from build123d import *

# Parameters (mm, degrees)
SKETCH1_R           = 29.337
BOSS_EXTRUDE1_DEPTH = 55.1942
SKETCH2_R           = 10.31875
SKETCH2_R_2         = 9.525
BOSS_EXTRUDE2_DEPTH = 3.175
SKETCH3_R           = 4.0005
BOSS_EXTRUDE3_DEPTH = 34.925
SKETCH4_R           = 2.0193
CUT_EXTRUDE1_DEPTH  = 12.7
CUT_EXTRUDE2_DEPTH  = 5.08
CUT_EXTRUDE3_DEPTH  = 2
FILLET1_R           = 0.127


with BuildPart() as part:
    # Sketch1 → Boss-Extrude1 (new body)
    with BuildSketch(Plane.XY):
        Circle(SKETCH1_R)
    extrude(amount=BOSS_EXTRUDE1_DEPTH)

    # Sketch2 → Boss-Extrude2 (add)
    with BuildSketch(Plane.XY.offset(55.1942)):
        Circle(SKETCH2_R)
        Circle(SKETCH2_R_2, mode=Mode.SUBTRACT)
    extrude(amount=BOSS_EXTRUDE2_DEPTH)

    # Sketch3 → Boss-Extrude3 (add)
    with BuildSketch(Plane.XY.offset(55.1942)):
        Circle(SKETCH3_R)
    extrude(amount=BOSS_EXTRUDE3_DEPTH)

    # Sketch4 → Cut-Extrude1 (cut)
    with BuildSketch(Plane.XY.offset(55.1942)):
        with Locations((17.960512242, -17.960512242)):
            Circle(SKETCH4_R)
        with Locations((-17.960512242, -17.960512242)):
            Circle(SKETCH4_R)
        with Locations((-17.960512242, 17.960512242)):
            Circle(SKETCH4_R)
        with Locations((17.960512242, 17.960512242)):
            Circle(SKETCH4_R)
    extrude(amount=-CUT_EXTRUDE1_DEPTH, mode=Mode.SUBTRACT)

    # Sketch5 → Cut-Extrude2 (cut)
    with BuildSketch(Plane(origin=(0, 29.337, 0), x_dir=(1, 0, 0), z_dir=(0, 1, 0))):
        with BuildLine():
            Line((12.7, -52.0192), (-12.7, -52.0192))
            ThreePointArc((-12.7, -52.0192), (-15.875, -48.8442), (-12.7, -45.6692))
            Line((-12.7, -45.6692), (12.7, -45.6692))
            ThreePointArc((12.7, -45.6692), (15.875, -48.8442), (12.7, -52.0192))
        make_face()
    extrude(amount=-CUT_EXTRUDE2_DEPTH, mode=Mode.SUBTRACT)

    # Sketch6 → Cut-Extrude3 (cut)
    with BuildSketch(Plane(origin=(0, 4.0005, 0), x_dir=(1, 0, 0), z_dir=(0, 1, 0))):
        with BuildLine():
            Line((0.99949, -65.71869), (0.99949, -85.21827))
            ThreePointArc((0.99949, -85.21827), (0, -86.21776), (-0.99949, -85.21827))
            Line((-0.99949, -85.21827), (-0.99949, -65.71869))
            ThreePointArc((-0.99949, -65.71869), (0, -64.7192), (0.99949, -65.71869))
        make_face()
    extrude(amount=-CUT_EXTRUDE3_DEPTH, mode=Mode.SUBTRACT)

    # Fillet1
    fillet1_edges = [part.edges().sort_by_distance(p)[0] for p in [
        (-4.0005, 0, 90.1192),
    ]]
    fillet(fillet1_edges, radius=FILLET1_R)


solid = part.part
Build history of the part. All positions in model axes, mm. A direction names the side the tool comes from. Coordinates: 2 decimals unless noted, no trailing zeros. Order: outer loops, then holes, each group sorted by start corner. A loop starts at its lowest first (then second) coordinate and runs counter-clockwise, first axis right, second up. Notation, with made-up numbers: (74.5, -32.75) - (108.5, -32.75) arc R37 ccw to (108.5, 4.25) - close; hole circle Ø1 at (-37.5, 25). An arc over 180 degrees is marked (long way). Put each result on its own line as item: value.
1. Pull direction Z, two halves, no side cores. Call faces 4 (the face through (17.698, 19.963, 48.933)), 5 (the face through (13, 0, 55.194)), 6 (the face through (-15.7, 24.6, 47.8)): pulls with the +Z half, pulls with the -Z half, needs draft (parallel to the pull), parting line crosses it, or undercut.
Answer sheet:
face 4: needs draft
face 5: pulls with the +Z half
face 6: undercut
2. Probe line 1 along Y through (x, z) = (0, 56) (1 decimal); line 2 along Z through (x, y) = (4, 25.5); line 3 along Y through (x, z) = (-1.5, 55.5). List the from-to ranges inside material, lowest first. Write a range as [from, to].
Answer sheet:
line 1: y = [-10.3, -9.5], [-4, 4], [9.5, 10.3]
line 2: z = [0, 45.67], [52.02, 55.19]
line 3: y = [-10.21, -9.41], [-3.71, 3.71], [9.41, 10.21]
3. Saw through at B-B (x = 7). Write the cut outline in (y, z), and give its area (3 significant figures).
Answer sheet:
outline: (-28.49, 0) - (28.49, 0) - (28.49, 45.67) - (24.26, 45.67) - (24.26, 52.02) - (28.49, 52.02) - (28.49, 55.19) - (7.58, 55.19) - (7.58, 58.37) - (6.46, 58.37) - (6.46, 55.19) - (-6.46, 55.19) - (-6.46, 58.37) - (-7.58, 58.37) - (-7.58, 55.19) - (-28.49, 55.19) - close
area: 3,130 mm^2
4. Tool access for faces 1 (the face through (-2.237, -10.073, 56.759)), 2 (the face through (0, 0, 90.119)), 3 (the face through (0, 2, 75)): list every direction of +Z, -Z, +X, -X, +Y, -Y with a clear straight run to the whole face (end or side of a thin tool).
Answer sheet:
face 1: +Z
face 2: +Z, +X, -X, +Y, -Y
face 3: +Y
5. Saw through at D-D (z = 30). Write the cut outline in (x, y), and give its area (3 significant figures).
Answer sheet:
outline: circle Ø58.67 at (0, 0)
area: 2,700 mm^2
6. Saw through at C-C (z = 53.5). Write the cut outline in (x, y).
Answer sheet:
outline: circle Ø58.67 at (0, 0); hole circle Ø4.04 at (-17.96, -17.96); hole circle Ø4.04 at (-17.96, 17.96); hole circle Ø4.04 at (17.96, -17.96); hole circle Ø4.04 at (17.96, 17.96)
7. Drop flat-ended pins along their axis: P1, Ø3.5, axis at x = -17.96, y = -17.96, coming from the +Z side; P2, Ø1.5, axis at y = -8, z = 39, coming from the +X side; P3, Ø6, axis at x = 7, y = -2.5, coming from the +Z side. Give the stop position or say it passes through.
Answer sheet:
P1: stops at z = 42.49
P2: stops at x = 28.43
P3: stops at z = 58.37
